Answer from the drawing. Dimensions are ordinates in mm from the lowest x, y and z of the part. Round coordinates to 2 decimals unless told otherwise and drop trailing zeros. Loops run counter-clockwise (first coordinate to the right, second up) from the corner with the lowest first, then second, coordinate; pieces in that order, holes last. Notation, with made-up numbers: (73, 22.25) - (112, 22.25) arc R13 cw to (112, 45.25) - close; hole circle Ø2 at (-7.75, 10.5). An arc over 180 degrees is marked (long way). Use CSV: the item, a comma, the result in double quotes. Start each with the question number.
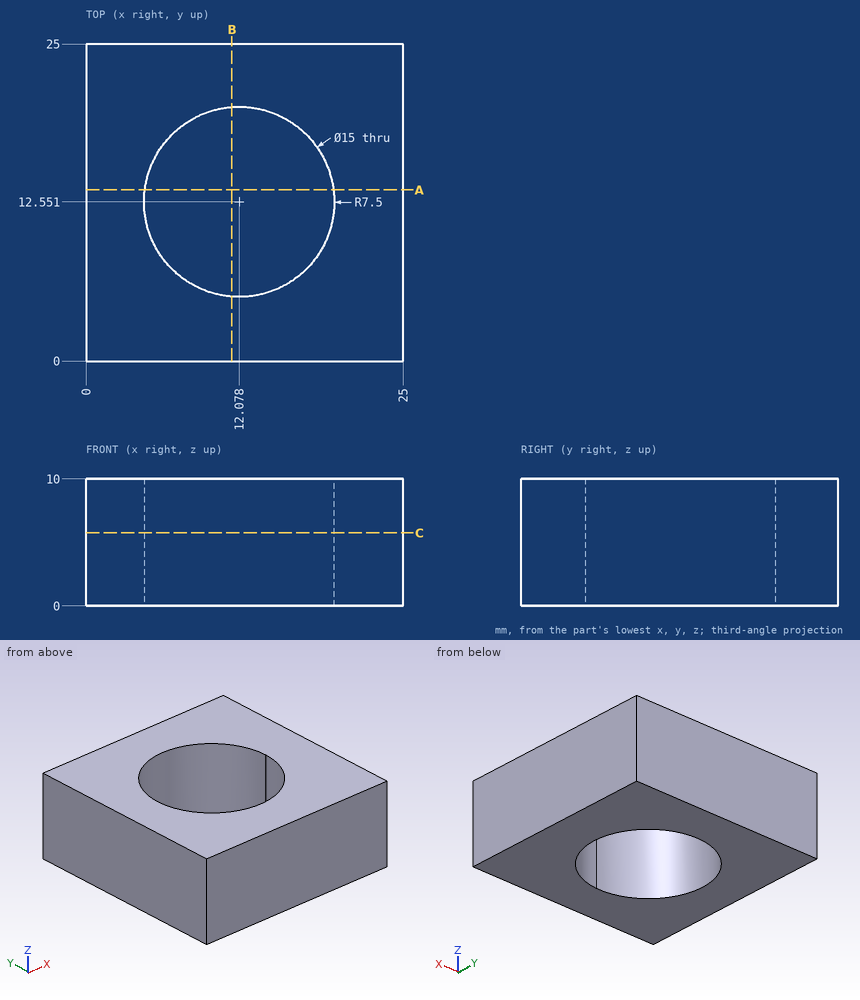
Item 1: A cutting plane is placed at C-C (z = 5.75). Determine the outline of the cut face in (x, y), plus the area to 3 significant figures.
Item 2: A cutting plane is placed at B-B (x = 11.5). Determine the outline of the cut face in (y, z), plus the area to 3 significant figures.
Item 3: A cutting plane is placed at A-A (y = 13.5). Determine the outline of the cut face in (x, z).
Item 4: Find the intervals of material crossed by probe 1 along X at (y, z) = (8.75, 3.25) (1 decimal); probe 2 along X at (y, z) = (13.25, 9.5) (1 decimal); probe 3 along Y at (x, z) = (9.25, 4) (1 decimal), in increasing order. Write a range as [from, to].
Item 5: This flat-tipped pin is pushed along its axis until it touches: pin 1 Ø13.5 at (x, y) = (12.08, 12.55) entering from +Z. Where does it stop, or does it pass through?
Result sheet:
1,outline,"(0, 0) - (25, 0) - (25, 25) - (0, 25) - close; hole (19.58, 12.5) arc R7.5 ccw to (19.58, 12.55) arc R7.5 ccw (long way) to start"
1,area,"448 mm^2"
2,outline,"(0, 0) - (5.07, 0) - (5.07, 10) - (0, 10) - close; (20.03, 0) - (25, 0) - (25, 10) - (20.03, 10) - close"
2,area,"100 mm^2"
3,outline,"(0, 0) - (4.64, 0) - (4.64, 10) - (0, 10) - close; (19.52, 0) - (25, 0) - (25, 10) - (19.52, 10) - close"
4,probe 1,"[0, 5.6], [18.5, 25]"
4,probe 2,"[0, 4.6], [19.5, 25]"
4,probe 3,"[0, 5.6], [19.5, 25]"
5,pin 1,"through"
